Part model, mm, in its own coordinate system. A direction names the side the tool comes from. Give positions to 0.01 mm unless a question says otherwise; leave off trailing zeros. Order: outer loops, then holes, each group sorted by start corner. A loop starts at its lowest first (then second) coordinate and runs counter-clockwise, first axis right, second up. Notation, with made-up numbers: (39, 22) - (83, 22) arc R36 cw to (83, 57) - close; hole circle Ø8 at (-12, 15). An arc over 180 degrees is marked (long way). One line per item, written item: value.
Autodesk Inventor part; units mm, degrees
ref_plane "YZ Plane" through (0, 0, 0) normal (1, 0, 0) x (0, 1, 0)
ref_plane "XZ Plane" through (0, 0, 0) normal (0, 1, 0) x (-1, 0, 0)
ref_plane "XY Plane" through (0, 0, 0) normal (0, 0, 1) x (1, 0, 0)
sketch "Sketch1" plane through (0, 0, 0) normal (0, 0, 1) x (1, 0, 0)
  circle A0 centre (0, 0) radius 11
  circle A1 centre (0, 0) radius 4
  dimension "d0" = 22
  dimension "d1" = 8
extrude "Extrusion1" add sketch "Sketch1" along normal blind 7
sketch "Sketch2" plane through (0, 0, 7) normal (0, 0, 1) x (1, 0, 0)
  circle A0 centre (0, 0) radius 5
  circle A1 centre (0, 0) radius 10
  circle A2 centre (0, 0) radius 11
  circle A3 centre (0, 0) radius 4
  dimension "d4" = 1
  dimension "d5" = 1
extrude "Extrusion2" cut sketch "Sketch2" against normal blind 0.25 contours A1
sketch "Sketch3" plane through (0, 0, 0) normal (0, 0, -1) x (-1, 0, 0)
  circle A0 centre (0, 0) radius 10
  circle A1 centre (0, 0) radius 5
extrude "Extrusion3" cut sketch "Sketch3" against normal blind 0.25
chamfer "Chamfer1" distance 0.25 angle 45 2 edges at (-11, 0, 7) (-11, 0, 0)
properties part number "bearing_22x8x7"
1) Drill centre lines: line 1 along Y through (x, z) = (0, 6.9); line 2 along Y through (x, z) = (0, 2.75); line 3 along Y through (x, z) = (0, 0.2). Where is each one in solid material? Low to high. Write a range as from..to.
Outcome:
line 1: y = -10.85..-10, -5..-4, 4..5, 10..10.85
line 2: y = -11..-4, 4..11
line 3: y = -10.95..-10, -5..-4, 4..5, 10..10.95
2) Cut at A-A, the plane x = 0. Give the cut face in (y, z), then the cut area to 3 significant figures.
Outcome:
outline: (-11, 0.25) - (-10.75, 0) - (-10, 0) - (-10, 0.25) - (-5, 0.25) - (-5, 0) - (-4, 0) - (-4, 7) - (-5, 7) - (-5, 6.75) - (-10, 6.75) - (-10, 7) - (-10.75, 7) - (-11, 6.75) - close; (4, 0) - (5, 0) - (5, 0.25) - (10, 0.25) - (10, 0) - (10.75, 0) - (11, 0.25) - (11, 6.75) - (10.75, 7) - (10, 7) - (10, 6.75) - (5, 6.75) - (5, 7) - (4, 7) - close
area: 92.9 mm^2
3) Mould opens along X. For faces 1 (the flat face through (3, -10, 7)), 2 (the cylindrical face through (-0.867, 3.905, 3.451)), 3 (the cylindrical face through (-2.38, 10.74, 3.45)) say: released by +X, released by -X, zero draft, split by the parting line, or undercut.
Outcome:
face 1: zero draft
face 2: undercut
face 3: split by the parting line
4) Pin check, flat tips, straight feed: pin 1 (4 mm diameter, centred on x = -7, y = 7.5, fed in from -Z); pin 2 (3 mm diameter, centred on x = -2.5, z = 5.5, fed in from -Y); pin 3 (4 mm diameter, centred on y = 6.5, z = 5, fed in from +X); pin 4 (1 mm diameter, centred on x = -3, y = -7.5, fed in from -Z). Stop position of each tip, or through.
Outcome:
pin 1: stops at z = 0
pin 2: stops at y = -10.95
pin 3: stops at x = 10.04
pin 4: stops at z = 0.25
5) Which spindle directions (+Z, -Z, +X, -X, +Y, -Y) get a long thin tool onto all of the face, cutting with end or side? Do faces 4 (the flat face through (3, -10, 0)), 5 (the flat face through (-2, 5, 0.25)), 6 (the flat face through (2, 5, 6.75)). Say none if no direction does.
Outcome:
face 4: -Z, +X, -X, +Y, -Y
face 5: -Z
face 6: +Z
6) Cut at C-C, the plane z = 1.25. Give the cut face in (x, y), then the cut area to 3 significant figures.
Outcome:
outline: circle Ø22 at (0, 0); hole circle Ø8 at (0, 0)
area: 330 mm^2
